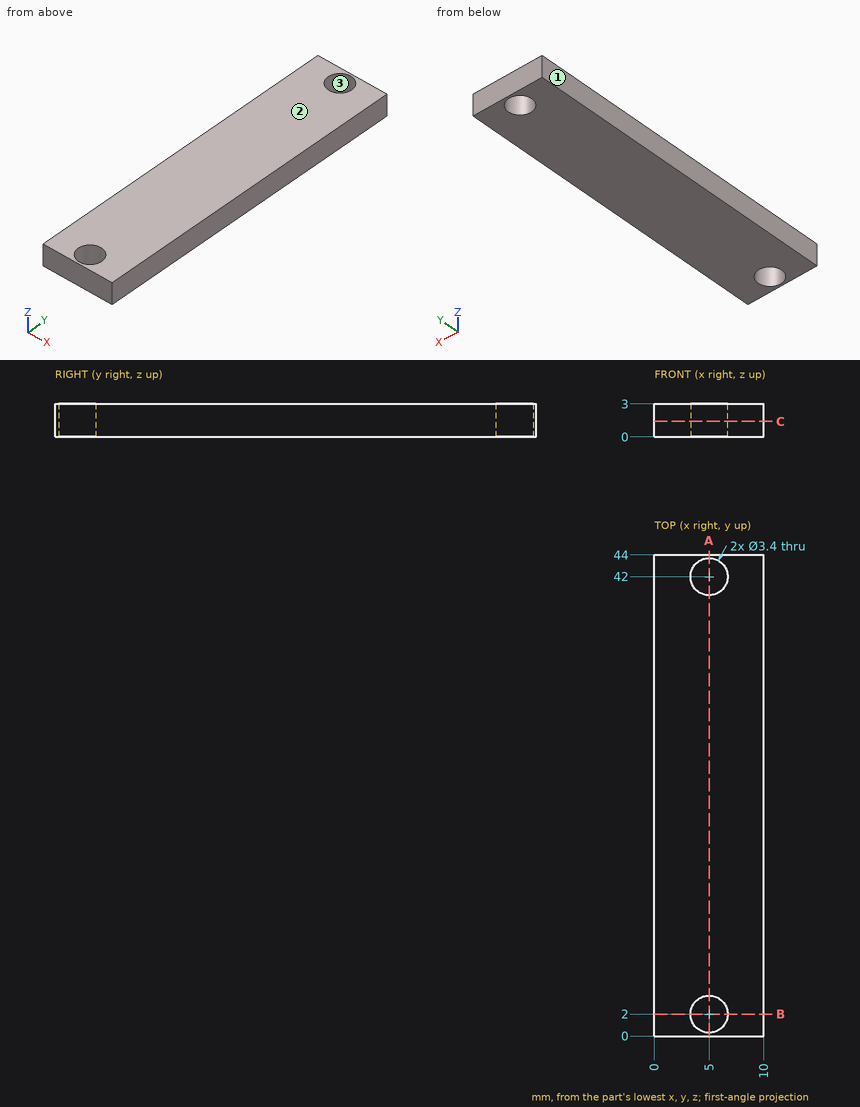
Job drawing, mm, ordinate dimensions from the low corner. One solid piece. Give positions to 0.01 mm unless a question says otherwise; leave off trailing zeros. Loops run counter-clockwise (first coordinate to the right, second up) from the corner with the lowest first, then second, coordinate; pieces in that order, holes last. Notation, with made-up numbers: (65, 8) -> (87, 8) arc R12 cw to (87, 16) -> close; hole circle Ø6 at (16, 30). An arc over 180 degrees is marked (long way). Write each question's results on one line, items separated by ' | '. Start each with the question number.
Q1. Band-saw the part on A-A on x = 5. List the corners of the cut face in (y, z), plus the area to 3 significant figures.
Q2. Wall check: L1, parallel to Y at x = 5, z = 1.45; L2, parallel to X at y = 2, z = 1.6; L3, parallel to Y at x = 4, z = 2.6. Give the ranges that are in metal, low to high.
Q3. Band-saw the part on B-B on y = 2. List the corners of the cut face in (x, z).
Q4. Pull direction X, two halves, no side cores. Call the marked faces 1, 2 and 3: +X half, -X half, draft (parallel to the pull), parting line (faces both ways), or undercut.
Q5. Band-saw the part on C-C on z = 1.4. List the corners of the cut face in (x, y).
Q6. Pin check, flat tip, straight feed: P1, Ø3, axis at x = 5, y = 2, coming from the +Z side. Stop position of the tip, or through.
Results are:
1) outline: (0, 0) -> (0.3, 0) -> (0.3, 3) -> (0, 3) -> close; (3.7, 0) -> (40.3, 0) -> (40.3, 3) -> (3.7, 3) -> close; (43.7, 0) -> (44, 0) -> (44, 3) -> (43.7, 3) -> close | area: 112 mm²
2) L1: y = 0 to 0.3, 3.7 to 40.3, 43.7 to 44 | L2: x = 0 to 3.3, 6.7 to 10 | L3: y = 0 to 0.63, 3.37 to 40.63, 43.37 to 44
3) outline: (0, 0) -> (3.3, 0) -> (3.3, 3) -> (0, 3) -> close; (6.7, 0) -> (10, 0) -> (10, 3) -> (6.7, 3) -> close
4) face 1: -X half | face 2: draft | face 3: undercut
5) outline: (0, 0) -> (10, 0) -> (10, 44) -> (0, 44) -> close; hole circle Ø3.4 at (5, 2); hole circle Ø3.4 at (5, 42)
6) P1: passes through
